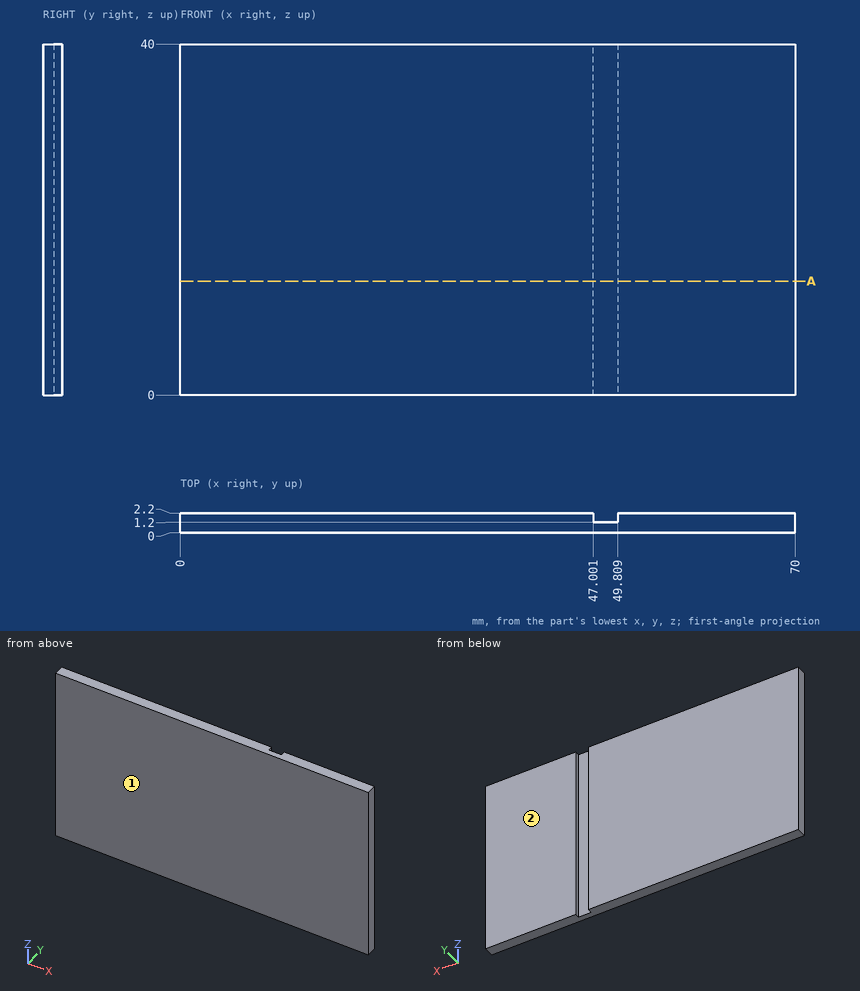
Design review of the part shown in the three views and the two pictorial views. Dimensions are in mm from the part's minimum x, y and z. Round coordinates to 2 decimals unless told otherwise and drop trailing zeros. Write each loop counter-clockwise with the first axis right and the second up, starting at its lowest first coordinate (ties: lowest second). Pieces come first, ordered by that corner, then holes. Notation, with made-up numbers: (54, -29.5) -> (72, -29.5) arc R31 cw to (72, 3.5) -> close; hole circle Ø6 at (22, -15.75). An arc over 180 degrees is marked (long way). One line per question, with ' | ' between items. Start each with the question number.
1) Wall thickness on line 1 along X through (y, z) = (1.7, 6.5); line 2 along Y through (x, z) = (49, 2.5): over which ranges is each line inside the solid? List them lowest first.
2) For pin 1 Ø0.8 at (x, z) = (49, 15) entering from +Y, flat-tipped, find the tip position at first contact; note if it passes through.
3) Add section A-A (z = 13). Write out the cut boundary in (x, y), and give its area (3 significant figures).
4) Mouldability with a two-part tool opening along Y and no side actions: class the marked faces 1 and 2 as +Y half, -Y half, draft (parallel to the pull), parting line (faces both ways), or undercut.
Reported:
1) line 1: x = 0 to 47, 49.81 to 70 | line 2: y = 0 to 1.2
2) pin 1: stops at y = 1.2
3) outline: (0, 0) -> (70, 0) -> (70, 2.2) -> (49.81, 2.2) -> (49.81, 1.2) -> (47, 1.2) -> (47, 2.2) -> (0, 2.2) -> close | area: 151 mm²
4) face 1: -Y half | face 2: +Y half
